Can you work these out from the model? Positions are in its coordinate system, mm. A direction names the side the tool comes from. Give positions to 0.01 mm unless a question says otherwise; leave off trailing zeros. Write each loop counter-clockwise with the first axis right and the second up, starting at its lowest first coordinate (ties: lowest second). Pieces come first, ordered by that corner, then holes.
```python
from build123d import *

# Parameters (mm, degrees)
SKETCH_W      = 65
SKETCH_H      = 29
PAD_DEPTH     = 2
SKETCH002_W   = 69
SKETCH002_H   = 33
PAD001_DEPTH  = 2
SKETCH003_W   = 20
SKETCH003_H   = 20
SKETCH003_W_2 = 26
SKETCH003_H_2 = 19
POCKET_DEPTH  = 4.001


with BuildPart() as part:
    # Sketch → Pad (new body)
    with BuildSketch(Plane.XY):
        Rectangle(SKETCH_W, SKETCH_H)
    extrude(amount=PAD_DEPTH)

    # Sketch002 (on Face5 of Pad) → Pad001 (join)
    with BuildSketch(Plane(origin=(0, 0, 0), x_dir=(1, 0, 0), z_dir=(0, 0, -1))):
        Rectangle(SKETCH002_W, SKETCH002_H)
    extrude(amount=PAD001_DEPTH)

    # Sketch003 (on Face11 of Pad001) → Pocket (cut, through all)
    with BuildSketch(Plane.XY.offset(2)):
        with Locations((-16, 0.2)):
            Rectangle(SKETCH003_W, SKETCH003_H)
        with Locations((12.2, -0.4)):
            Rectangle(SKETCH003_W_2, SKETCH003_H_2)
    extrude(amount=-POCKET_DEPTH, mode=Mode.SUBTRACT)


solid = part.part
```
1) Suppose I cut it at D-D on y = -11.5. Write out the boundary of the cut face in (x, z).
Values follow:
outline: (-34.5, -2) - (34.5, -2) - (34.5, 0) - (32.5, 0) - (32.5, 2) - (-32.5, 2) - (-32.5, 0) - (-34.5, 0) - close
2) Suppose I cut it at A-A on x = -22.5. Write out the boundary of the cut face in (y, z), plus the area to 3 significant figures.
Values follow:
outline: (-16.5, -2) - (-9.8, -2) - (-9.8, 2) - (-14.5, 2) - (-14.5, 0) - (-16.5, 0) - close; (10.2, -2) - (16.5, -2) - (16.5, 0) - (14.5, 0) - (14.5, 2) - (10.2, 2) - close
area: 44.0 mm2
3) If we mould it in two halves opening along X, with no side actions, what happens to faces 1 (the face through (0, 14.5, 1)), 2 (the face through (34.5, 0, -1)), 3 (the face through (-16, 10.2, 0)), 4 (the face through (-6, 0, 0))? For each: +X half, -X half, draft (parallel to the pull), parting line (faces both ways), or undercut.
Values follow:
face 1: draft
face 2: +X half
face 3: undercut
face 4: undercut
4) Please list where these lines run through material, in increasing order: L1, parallel to X at y = 7, z = -1.65; L2, parallel to X at y = 7, z = 0.8; L3, parallel to Y at x = -24.5, z = -1.05.
Values follow:
L1: x = -34.5 to -26, -6 to -0.8, 25.2 to 34.5
L2: x = -32.5 to -26, -6 to -0.8, 25.2 to 32.5
L3: y = -16.5 to -9.8, 10.2 to 16.5
5) Suppose I cut it at B-B on z = 0.6. Write out the boundary of the cut face in (x, y).
Values follow:
outline: (-32.5, -14.5) - (32.5, -14.5) - (32.5, 14.5) - (-32.5, 14.5) - close; hole (-26, -9.8) - (-6, -9.8) - (-6, 10.2) - (-26, 10.2) - close; hole (-0.8, -9.9) - (25.2, -9.9) - (25.2, 9.1) - (-0.8, 9.1) - close
6) For pin 1 Ø1 at (x, z) = (-10, 1) entering from -Y; pin 2 Ø1.5 at (y, z) = (-13, 1) entering from -X; pin 3 Ø1.5 at (x, z) = (-13, 1.5) entering from +Y, each with a flat end and sliding along its axis, tell me the tip position at first contact or that it passes through.
Values follow:
pin 1: stops at y = -14.5
pin 2: stops at x = -32.5
pin 3: stops at y = 14.5
7) For faces 5 (the face through (0, -14.5, 1)), 6 (the face through (32.5, 0, 1)), 7 (the face through (12, -9.9, 0)), 8 (the face through (0, 10, 2)), 9 (the face through (-32.5, 0, 1)), which set-ups out of +Z, -Z, +X, -X, +Y, -Y let a thin tool reach every point of the face, with its end or its side?
Values follow:
face 5: +Z, +X, -X, -Y
face 6: +Z, +X, +Y, -Y
face 7: +Z, -Z
face 8: +Z, +X, -X, +Y, -Y
face 9: +Z, -X, +Y, -Y
8) Suppose I cut it at C-C on y = -4. Write out the boundary of the cut face in (x, z).
Values follow:
outline: (-34.5, -2) - (-26, -2) - (-26, 2) - (-32.5, 2) - (-32.5, 0) - (-34.5, 0) - close; (-6, -2) - (-0.8, -2) - (-0.8, 2) - (-6, 2) - close; (25.2, -2) - (34.5, -2) - (34.5, 0) - (32.5, 0) - (32.5, 2) - (25.2, 2) - close
